Geometry: see drawing. Coordinates: mm, zero at the bounding-box minimum. A direction names the side the tool comes from. Coordinates: 2 decimals unless noted, no trailing zeros. Write each loop counter-clockwise with the first axis right and the second up, starting at its lowest first coordinate (ties: lowest second). Pieces come first, ordered by that corner, then holes.
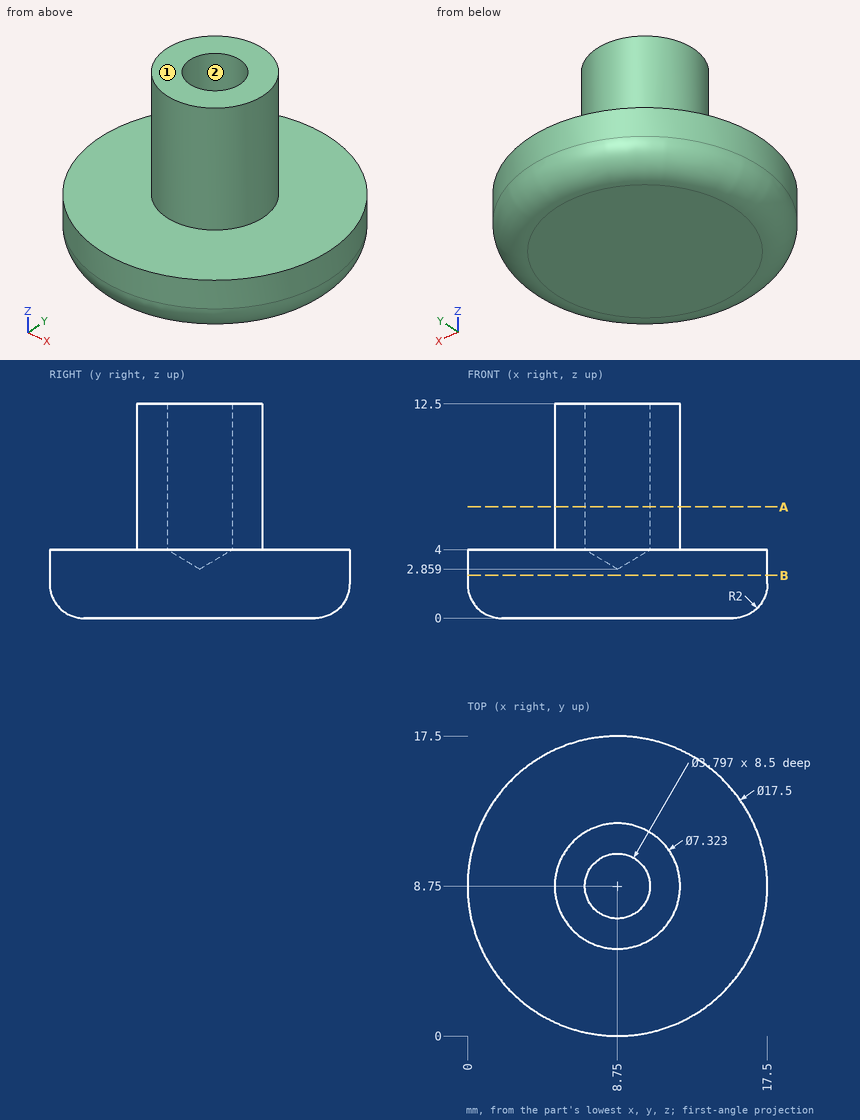
Item 1: Section A-A, the plane z = 6.5. Output: boundary loops of the cut face in (x, y), plus the area to 3 significant figures.
Derived:
outline: circle Ø7.32 at (8.75, 8.75); hole circle Ø3.8 at (8.75, 8.75)
area: 30.8 mm2
Item 2: Material intervals for probe 1 along Y at (x, z) = (8.75, 10.75); probe 2 along Z at (x, y) = (6.75, 5.25); probe 3 along X at (y, z) = (8, 6.25) (1 decimal), sorted ascending.
Derived:
probe 1: y = 5.09 to 6.85, 10.65 to 12.41
probe 2: z = 0 to 4
probe 3: x = 5.2 to 7, 10.5 to 12.3
Item 3: Section B-B, the plane z = 2.5. Output: boundary loops of the cut face in (x, y).
Derived:
outline: circle Ø17.5 at (8.75, 8.75)
Item 4: Set-up query: the marked faces 1 and 2. Return all of +Z, -Z, +X, -X, +Y, -Y with unobstructed straight access to the full face (end or side cutting, diameter ignored); none if empty.
Derived:
face 1: +Z, +X, -X, +Y, -Y
face 2: +Z
Item 5: Pin query (flat end, axial travel): pin 1 (4 mm diameter, centred on y = 2, z = 5.5, fed in from +X); pin 2 (1 mm diameter, centred on x = 3, z = 1.5, fed in from -Y) (1 decimal); pin 3 (1.5 mm diameter, centred on x = 12, z = 1.5, fed in from +Y). Return the tip coordinate at first contact, or that it passes through.
Derived:
pin 1: stops at x = 15.61
pin 2: stops at y = 1.8
pin 3: stops at y = 17.11
